Design review of the part shown in the three views and the two pictorial views. Dimensions are in mm from the part's minimum x, y and z. Give positions to 0.01 mm unless a question says otherwise; leave off trailing zeros. Loops run counter-clockwise (first coordinate to the right, second up) from the corner with the lowest first, then second, coordinate; pieces in that order, holes last. Notation, with made-up numbers: (-16.75, -25) -> (9.25, -25) arc R22 cw to (9.25, -4) -> close; hole circle Ø11 at (79, -28). An arc over 180 degrees is marked (long way). Use CSV: the item, a comma, the result in double quotes. Start each with the question number.
Item 1: We need section C-C (z = 36.5). State the section outline as (x, y) points, plus the area to 3 significant figures.
Item 2: Wall thickness on line 1 along X through (y, z) = (0.6, 5.5); line 2 along X through (y, z) = (1.6, 36.5); line 3 along X through (y, z) = (0.7, 21): over which ranges is each line inside the solid? List them lowest first. Write a range as from..to.
Item 3: We need section B-B (y = 1.35). State the section outline as (x, z) points.
Item 4: We need section A-A (x = 14.5). State the section outline as (y, z) points.
Item 5: Clearance check with flat-ended pins moving along their axes: pin 1 (1 mm diameter, centred on y = 0.5, z = 29.5, fed in from -X); pin 2 (0.6 mm diameter, centred on x = 20, y = 1, fed in from +Z); pin 3 (1 mm diameter, centred on y = 0.5, z = 3, fed in from +X). State where each tip first meets the part, or that it passes through.
Item 6: We need section D-D (x = 25). State the section outline as (y, z) points, plus the area to 3 significant figures.
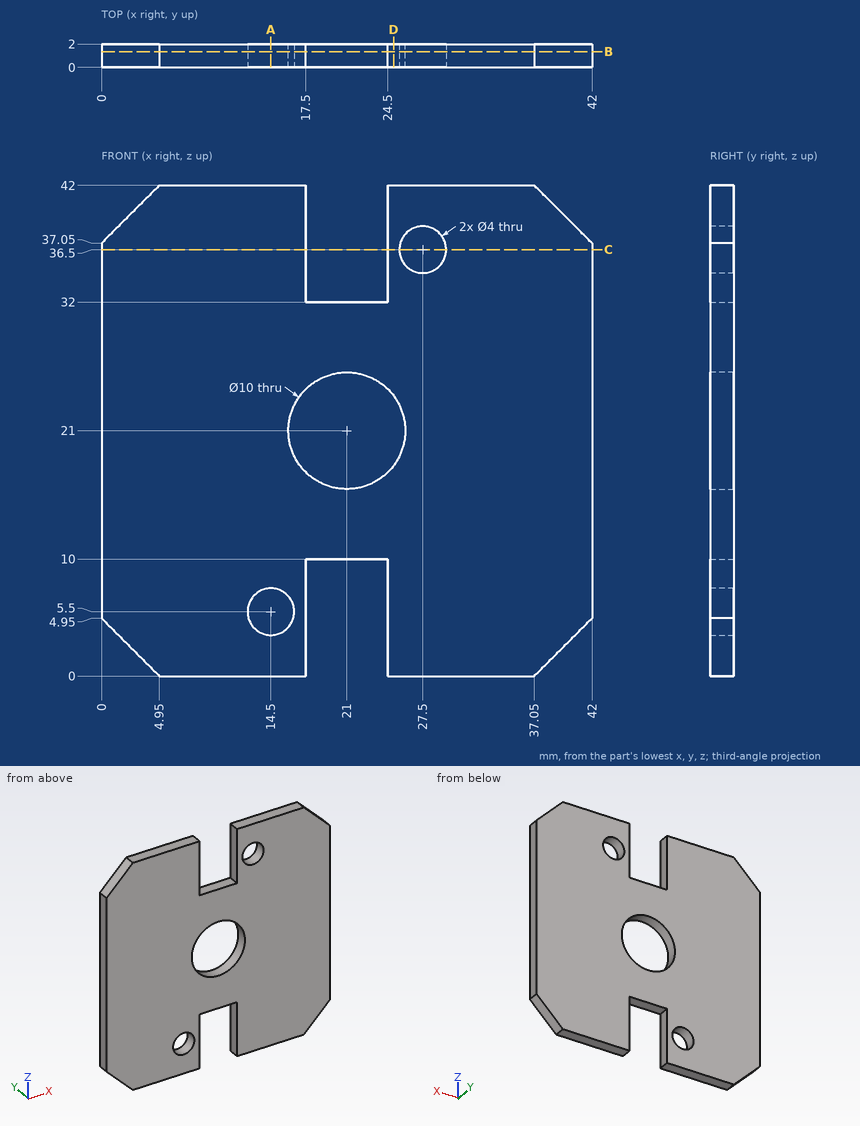
Results found:
1,outline,"(0, 0) -> (17.5, 0) -> (17.5, 2) -> (0, 2) -> close; (24.5, 0) -> (25.5, 0) -> (25.5, 2) -> (24.5, 2) -> close; (29.5, 0) -> (42, 0) -> (42, 2) -> (29.5, 2) -> close"
1,area,"62.0 mm²"
2,line 1,"0..12.5, 16.5..17.5, 24.5..42"
2,line 2,"0..17.5, 24.5..25.5, 29.5..42"
2,line 3,"0..16, 26..42"
3,outline,"(0, 4.95) -> (4.95, 0) -> (17.5, 0) -> (17.5, 10) -> (24.5, 10) -> (24.5, 0) -> (37.05, 0) -> (42, 4.95) -> (42, 37.05) -> (37.05, 42) -> (24.5, 42) -> (24.5, 32) -> (17.5, 32) -> (17.5, 42) -> (4.95, 42) -> (0, 37.05) -> close; hole circle Ø4 at (14.5, 5.5); hole circle Ø10 at (21, 21); hole circle Ø4 at (27.5, 36.5)"
4,outline,"(0, 0) -> (2, 0) -> (2, 3.5) -> (0, 3.5) -> close; (0, 7.5) -> (2, 7.5) -> (2, 42) -> (0, 42) -> close"
5,pin 1,"x = 0"
5,pin 2,"z = 32"
5,pin 3,"x = 40.55"
6,outline,"(0, 0) -> (2, 0) -> (2, 18) -> (0, 18) -> close; (0, 24) -> (2, 24) -> (2, 42) -> (0, 42) -> close"
6,area,"72.0 mm²"
